Here's how the part is built. I have some questions about the finished solid (model axes, mm). Round coordinates to 2 decimals unless told otherwise and drop trailing zeros. Order: outer loops, then holes, each group sorted by start corner. A loop starts at its lowest first (then second) coordinate and runs counter-clockwise, first axis right, second up. Notation, with made-up numbers: M -12.75,-38 L -7.75,-38 A21 cw -7.75,0 Z; hole C 23.25,17.25 d9. An arc over 180 degrees is marked long. Write item = value, one per line. Start each with the question number.
Item 1: I want a section at D-D, the plane z = -17.5. List the corners of the cut face in (x, y) for me.
Item 2: I'm going to push a flat-ended pin straight in: P1, Ø0.8, axis at x = -1, y = 67, coming from the +Z side. Where does the tip first touch, or does it pass through?
Item 3: I want a section at C-C, the plane y = 47.5. List the corners of the cut face in (x, z) for me.
Item 4: Please list where these lines run through material, in increasing order: L1, parallel to Y at x = -0.05, z = -32.25; L2, parallel to Y at x = -1.2, z = -32; L3, parallel to Y at x = -1, z = -33.
Item 5: I want a section at B-B, the plane x = -0.6. State how many separate pieces and enclosed holes the cut face has, plus the area to 3 significant figures.
Item 6: I want a section at A-A, the plane y = 25.8. List the corners of the cut face in (x, z) for me.
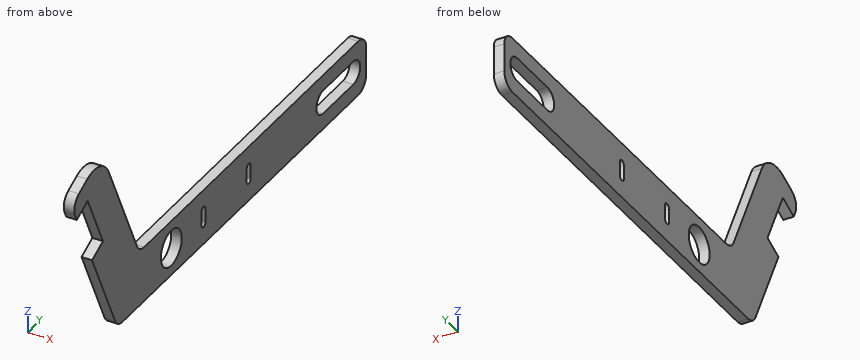
```python
from build123d import *

# Parameters (mm, degrees)
SKETCH1_R            = 2.6
BASE_FLANGE1_DEPTH   = 1.5
KEYING_DEPTH         = 10
FILLET1_R            = 2
FILLET2_R            = 4
JOG1_START           = -34.826317149
JOG1_DEPTH           = 8
JOG1_START_2         = -32.826317149
JOG1_2_DEPTH         = 0.3
JOG1_START_3         = -29.126317149
JOG1_3_DEPTH         = 0.3
JOG1_4_DEPTH         = 8
JOG1_START_4         = -13.5
JOG1_5_DEPTH         = 1.5
CUT_EXTRUDE1_START   = -13.5
CUT_EXTRUDE1_DEPTH   = 12
CUT_EXTRUDE1_START_2 = -1.5
CUT_EXTRUDE1_2_DEPTH = 1.5
CUT_EXTRUDE1_3_DEPTH = 1.5


with BuildPart() as part:
    # Base-Flange1: sheet metal written as solids
    # Sketch1 → Base-Flange1 (new body)
    with BuildSketch(Plane(origin=(0, 0, 0), x_dir=(0, 0, -1), z_dir=(1, 0, 0))):
        Polygon((34.826317149, 21.8), (34.826317149, 63.8), (26.826317149, 63.8), (26.826317149, 17.789661718), (6.95251297, 8.522354632), (9.826317149, 2.359461681), (10.460244542, 1), (34.826317149, 12.362086256), align=None)
        with Locations((30.826317149, 25.8)):
            Circle(SKETCH1_R, mode=Mode.SUBTRACT)
        with BuildLine():
            Line((32.526317149, 60.6), (32.526317149, 53.1))
            ThreePointArc((32.526317149, 53.1), (30.826317149, 51.4), (29.126317149, 53.1))
            Line((29.126317149, 53.1), (29.126317149, 60.6))
            ThreePointArc((29.126317149, 60.6), (30.826317149, 62.3), (32.526317149, 60.6))
        make_face(mode=Mode.SUBTRACT)
    extrude(amount=-BASE_FLANGE1_DEPTH)

    # Sketch6 → Keying (cut)
    with BuildSketch(Plane(origin=(0, 0, 0), x_dir=(0, 0, -1), z_dir=(1, 0, 0))):
        Polygon((21.335937987, 6.071419141), (20.068083201, 8.790342502), (11.911313118, 4.986778146), (13.179167903, 2.267854785), (16.260435533, 3.704673478), align=None)
    extrude(amount=-KEYING_DEPTH, mode=Mode.SUBTRACT)

    # Fillet1
    fillet1_edges = [part.edges().sort_by_distance(p)[0] for p in [
        (-0.75, 12.362086256, -34.826317149),
        (-0.75, 1, -10.460244542),
        (-0.75, 17.789661718, -26.826317149),
        (-0.75, 63.8, -26.826317149),
        (-0.75, 63.8, -34.826317149),
    ]]
    fillet(fillet1_edges, radius=FILLET1_R)

    # Fillet2
    fillet2_edges = [part.edges().sort_by_distance(p)[0] for p in [
        (-0.75, 8.522354632, -6.95251297),
    ]]
    fillet(fillet2_edges, radius=FILLET2_R)

    # Jog1: read off the stored shape, not the designer's step
    # Jog1 outline → Jog1 (cut)
    with BuildSketch(Plane.XY.offset(JOG1_START)):
        with BuildLine():
            Line((-1.5, 63.8), (-1.5, 34.716841062))
            ThreePointArc((-1.5, 34.716841062), (-0.408349934, 33.794859608), (0, 32.425553214))
            Line((0, 32.425553214), (0, 63.8))
            Line((0, 63.8), (-1.5, 63.8))
        make_face()
    extrude(amount=JOG1_DEPTH, mode=Mode.SUBTRACT)

    # Jog1 2 outline → Jog1 2 (add)
    with BuildSketch(Plane.XY.offset(JOG1_START_2)):
        with BuildLine():
            ThreePointArc((-1.5, 34.716841062), (-1.989225891, 34.872818996), (-2.5, 34.925553214))
            Line((-2.5, 34.925553214), (-11, 34.925553214))
            ThreePointArc((-11, 34.925553214), (-11.707106781, 35.218446433), (-12, 35.925553214))
            Line((-12, 35.925553214), (-12, 63.8))
            Line((-12, 63.8), (-13.5, 63.8))
            Line((-13.5, 63.8), (-13.5, 35.925553214))
            ThreePointArc((-13.5, 35.925553214), (-12.767766953, 34.157786261), (-11, 33.425553214))
            Line((-11, 33.425553214), (-2.5, 33.425553214))
            ThreePointArc((-2.5, 33.425553214), (-1.792893219, 33.132659995), (-1.5, 32.425553214))
            Line((-1.5, 32.425553214), (-1.5, 34.716841062))
        make_face()
    extrude(amount=JOG1_2_DEPTH)

    # Jog1 3 outline → Jog1 3 (add)
    with BuildSketch(Plane.XY.offset(JOG1_START_3)):
        with BuildLine():
            ThreePointArc((-1.5, 34.716841062), (-1.989225891, 34.872818996), (-2.5, 34.925553214))
            Line((-2.5, 34.925553214), (-11, 34.925553214))
            ThreePointArc((-11, 34.925553214), (-11.707106781, 35.218446433), (-12, 35.925553214))
            Line((-12, 35.925553214), (-12, 63.8))
            Line((-12, 63.8), (-13.5, 63.8))
            Line((-13.5, 63.8), (-13.5, 35.925553214))
            ThreePointArc((-13.5, 35.925553214), (-12.767766953, 34.157786261), (-11, 33.425553214))
            Line((-11, 33.425553214), (-2.5, 33.425553214))
            ThreePointArc((-2.5, 33.425553214), (-1.792893219, 33.132659995), (-1.5, 32.425553214))
            Line((-1.5, 32.425553214), (-1.5, 34.716841062))
        make_face()
    extrude(amount=JOG1_3_DEPTH)

    # Jog1 4 outline → Jog1 4 (add)
    with BuildSketch(Plane.XY.offset(JOG1_START)):
        with BuildLine():
            ThreePointArc((-1.5, 34.716841062), (-1.989225891, 34.872818996), (-2.5, 34.925553214))
            Line((-2.5, 34.925553214), (-11, 34.925553214))
            ThreePointArc((-11, 34.925553214), (-11.707106781, 35.218446433), (-12, 35.925553214))
            Line((-12, 35.925553214), (-12, 63.8))
            Line((-12, 63.8), (-13.5, 63.8))
            Line((-13.5, 63.8), (-13.5, 35.925553214))
            ThreePointArc((-13.5, 35.925553214), (-12.767766953, 34.157786261), (-11, 33.425553214))
            Line((-11, 33.425553214), (-2.5, 33.425553214))
            ThreePointArc((-2.5, 33.425553214), (-1.792893219, 33.132659995), (-1.5, 32.425553214))
            Line((-1.5, 32.425553214), (-1.5, 34.716841062))
        make_face()
    extrude(amount=JOG1_4_DEPTH)

    # Jog1 5 outline → Jog1 5 (cut)
    with BuildSketch(Plane.YZ.offset(JOG1_START_4)):
        with BuildLine():
            ThreePointArc((61.8, -26.826317149), (63.214213562, -27.412103587), (63.8, -28.826317149))
            Line((63.8, -28.826317149), (63.8, -26.826317149))
            Line((63.8, -26.826317149), (61.8, -26.826317149))
        make_face()
        with BuildLine():
            ThreePointArc((63.8, -32.826317149), (63.214213562, -34.240530711), (61.8, -34.826317149))
            Line((61.8, -34.826317149), (63.8, -34.826317149))
            Line((63.8, -34.826317149), (63.8, -32.826317149))
        make_face()
        with BuildLine():
            Line((60.6, -29.126317149), (53.1, -29.126317149))
            ThreePointArc((53.1, -29.126317149), (51.4, -30.826317149), (53.1, -32.526317149))
            Line((53.1, -32.526317149), (60.6, -32.526317149))
            ThreePointArc((60.6, -32.526317149), (62.3, -30.826317149), (60.6, -29.126317149))
        make_face()
    extrude(amount=JOG1_5_DEPTH, mode=Mode.SUBTRACT)

    # Cut-Extrude1: read off the stored shape, not the designer's step
    # Cut-Extrude1 outline → Cut-Extrude1 (cut)
    with BuildSketch(Plane(origin=(0, 0, 0), x_dir=(0, 0, -1), z_dir=(1, 0, 0)).offset(CUT_EXTRUDE1_START)):
        with BuildLine():
            Line((26.826317149, 31), (34.826317149, 31))
            Line((34.826317149, 31), (34.826317149, 61.8))
            ThreePointArc((34.826317149, 61.8), (34.240530711, 63.214213562), (32.826317149, 63.8))
            Line((32.826317149, 63.8), (28.826317149, 63.8))
            ThreePointArc((28.826317149, 63.8), (27.412103587, 63.214213562), (26.826317149, 61.8))
            Line((26.826317149, 61.8), (26.826317149, 31))
        make_face()
        with BuildLine():
            ThreePointArc((29.126317149, 60.6), (30.826317149, 62.3), (32.526317149, 60.6))
            Line((32.526317149, 60.6), (32.526317149, 53.1))
            ThreePointArc((32.526317149, 53.1), (30.826317149, 51.4), (29.126317149, 53.1))
            Line((29.126317149, 53.1), (29.126317149, 60.6))
        make_face(mode=Mode.SUBTRACT)
    extrude(amount=CUT_EXTRUDE1_DEPTH, mode=Mode.SUBTRACT)

    # Cut-Extrude1 2 outline → Cut-Extrude1 2 (cut)
    with BuildSketch(Plane(origin=(0, 0, 0), x_dir=(0, 0, -1), z_dir=(1, 0, 0)).offset(CUT_EXTRUDE1_START_2)):
        with BuildLine():
            ThreePointArc((29.826317149, 34.3), (29.326317149, 33.8), (29.826317149, 33.3))
            Line((29.826317149, 33.3), (31.826317149, 33.3))
            ThreePointArc((31.826317149, 33.3), (32.326317149, 33.8), (31.826317149, 34.3))
            Line((31.826317149, 34.3), (29.826317149, 34.3))
        make_face()
    extrude(amount=CUT_EXTRUDE1_2_DEPTH, mode=Mode.SUBTRACT)

    # Cut-Extrude1 3 outline → Cut-Extrude1 3 (add)
    with BuildSketch(Plane(origin=(0, 0, 0), x_dir=(0, 0, -1), z_dir=(1, 0, 0)).offset(CUT_EXTRUDE1_START_2)):
        with BuildLine():
            Line((26.826317149, 31), (34.826317149, 31))
            Line((34.826317149, 31), (34.826317149, 72.297787144))
            ThreePointArc((34.826317149, 72.297787144), (34.240530711, 73.712000706), (32.826317149, 74.297787144))
            Line((32.826317149, 74.297787144), (28.826317149, 74.297787144))
            ThreePointArc((28.826317149, 74.297787144), (27.412103587, 73.712000706), (26.826317149, 72.297787144))
            Line((26.826317149, 72.297787144), (26.826317149, 31))
        make_face()
        with BuildLine():
            ThreePointArc((29.826317149, 33.3), (29.326317149, 33.8), (29.826317149, 34.3))
            Line((29.826317149, 34.3), (31.826317149, 34.3))
            ThreePointArc((31.826317149, 34.3), (32.326317149, 33.8), (31.826317149, 33.3))
            Line((31.826317149, 33.3), (29.826317149, 33.3))
        make_face(mode=Mode.SUBTRACT)
        with BuildLine():
            Line((29.826317149, 45.548893572), (31.826317149, 45.548893572))
            ThreePointArc((31.826317149, 45.548893572), (32.326317149, 45.048893572), (31.826317149, 44.548893572))
            Line((31.826317149, 44.548893572), (29.826317149, 44.548893572))
            ThreePointArc((29.826317149, 44.548893572), (29.326317149, 45.048893572), (29.826317149, 45.548893572))
        make_face(mode=Mode.SUBTRACT)
        with BuildLine():
            Line((29.126317149, 63.597787144), (29.126317149, 71.097787144))
            ThreePointArc((29.126317149, 71.097787144), (30.826317149, 72.797787144), (32.526317149, 71.097787144))
            Line((32.526317149, 71.097787144), (32.526317149, 63.597787144))
            ThreePointArc((32.526317149, 63.597787144), (30.826317149, 61.897787144), (29.126317149, 63.597787144))
        make_face(mode=Mode.SUBTRACT)
    extrude(amount=CUT_EXTRUDE1_3_DEPTH)


solid = part.part
```
Filled in:
q1.outline = M -1.5,7.59 L 0,7.59 L 0,13.44 L -1.5,13.44 Z
q2.P1 = -26.83
q3.outline = M -1.5,-34.83 L 0,-34.83 L 0,-26.83 L -1.5,-26.83 Z
q4.L1 = 11.16 to 23.62, 27.98 to 33.53, 34.07 to 44.78, 45.31 to 62.67, 72.03 to 74.3
q4.L2 = 11.04 to 23.48, 28.12 to 33.33, 34.27 to 44.58, 45.52 to 62.37, 72.33 to 74.3
q4.L3 = 11.51 to 24.37, 27.23 to 74.29
q5.separate_pieces = 1
q5.enclosed_holes = 4
q5.area = 582 mm^2
q6.outline = M -1.5,-34.83 L 0,-34.83 L 0,-33.43 L -1.5,-33.43 Z; M -1.5,-28.23 L 0,-28.23 L 0,-26.83 L -1.5,-26.83 Z
